Input: part model. Units: mm. Frame: model coordinates. Face numbers are marked on the shaded views. Coordinates: 2 decimals unless noted, no trailing zeros. Order: outer loops, then holes, each group sorted by start corner. A loop starts at its lowest first (then second) coordinate and runs counter-clockwise, first axis right, second up. Notation, with made-up numbers: (-14.75, 82) -> (-3.75, 82) arc R25 cw to (-3.75, 115) -> close; hole circle Ø5 at (28.25, 84). An arc over 180 degrees is marked (long way). Use CSV: the item, a comma, the result in double quotes. Start each with the question number.
```python
from build123d import *

# Parameters (mm, degrees)
SKETCH1_R               = 50.8
BOSS_EXTRUDE1_DEPTH     = 6.35
SKETCH2_R               = 3.175
CUT_EXTRUDE1_DEPTH      = 2.286
SKETCH3_R               = 3.175
CUT_EXTRUDE2_DEPTH      = 1
CUT_EXTRUDE2_DEPTH_BACK = 7.35
SKETCH4_R               = 1.5875
CUT_EXTRUDE3_DEPTH      = 7.35
CHAMFER1_SIZE           = 0.762
FILLET1_R               = 1.27
SKETCH5_R               = 48
SKETCH5_R_2             = 46
BOSS_EXTRUDE2_DEPTH     = 6.35


with BuildPart() as part:
    # Sketch1 → Boss-Extrude1 (new body)
    with BuildSketch(Plane(origin=(0, 0, 0), x_dir=(1, 0, 0), z_dir=(0, 1, 0))):
        Circle(SKETCH1_R)
    extrude(amount=BOSS_EXTRUDE1_DEPTH)

    # Sketch2 → Cut-Extrude1 (cut)
    with BuildSketch(Plane(origin=(0, 6.35, 0), x_dir=(1, 0, 0), z_dir=(0, 1, 0))):
        with Locations((-22.225, -38.494829198)):
            Circle(SKETCH2_R)
        with Locations((-22.225, 38.494829198)):
            Circle(SKETCH2_R)
        with Locations((44.45, 0)):
            Circle(SKETCH2_R)
    extrude(amount=-CUT_EXTRUDE1_DEPTH, mode=Mode.SUBTRACT)

    # Sketch3 → Cut-Extrude2 (cut, two sides)
    with BuildSketch(Plane(origin=(0, 6.35, 0), x_dir=(1, 0, 0), z_dir=(0, 1, 0))) as cut_extrude2_sk:
        Circle(SKETCH3_R)
    extrude(amount=CUT_EXTRUDE2_DEPTH, mode=Mode.SUBTRACT)
    extrude(cut_extrude2_sk.sketch, amount=-CUT_EXTRUDE2_DEPTH_BACK, mode=Mode.SUBTRACT)

    # Sketch4 → Cut-Extrude3 (cut, through all)
    with BuildSketch(Plane.XZ):
        with Locations((50.8, 0)):
            Circle(SKETCH4_R)
        with Locations((-25.4, 43.994090512)):
            Circle(SKETCH4_R)
        with Locations((-25.4, -43.994090512)):
            Circle(SKETCH4_R)
    extrude(amount=-CUT_EXTRUDE3_DEPTH, mode=Mode.SUBTRACT)

    # Chamfer1
    chamfer1_edges = [part.edges().sort_by_distance(p)[0] for p in [
        (25.4, 0, -43.994090512),
        (-50.8, 0, 0),
        (25.4, 0, 43.994090512),
        (25.4, 6.35, -43.994090512),
        (-50.8, 6.35, 0),
        (25.4, 6.35, 43.994090512),
    ]]
    chamfer(chamfer1_edges, length=CHAMFER1_SIZE)

    # Fillet1
    fillet1_edges = [part.edges().sort_by_distance(p)[0] for p in [
        (-24.012950162, 3.175, 44.766262124),
        (-26.76224515, 3.175, 43.178955922),
        (50.775195313, 3.175, -1.587306202),
        (50.775195313, 3.175, 1.587306202),
        (-24.012950162, 3.175, -44.766262124),
        (-26.76224515, 3.175, -43.178955922),
    ]]
    fillet(fillet1_edges, radius=FILLET1_R)

    # Sketch5 → Boss-Extrude2 (add)
    with BuildSketch(Plane.XZ):
        Circle(SKETCH5_R)
        Circle(SKETCH5_R_2, mode=Mode.SUBTRACT)
    extrude(amount=BOSS_EXTRUDE2_DEPTH)


solid = part.part
```
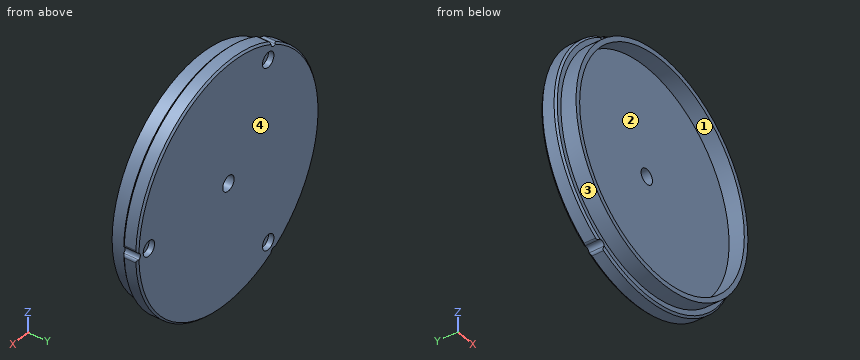
1. Contact query for flat-ended pins moving along their axis: P1, Ø3, axis at x = -22.5, z = 38.5, coming from the +Y side; P2, Ø1.5, axis at y = -1.5, z = 13, coming from the -X side; P3, Ø1.5, axis at x = 3.5, y = 0.5, coming from the +Z side. Output: stop coordinate, or through.
2. Section B-B on x = 0. Return loops of the section in (y, z) (3 decimals).
3. Material intervals for line 1 along X through (y, z) = (4.8, 0) (1 decimal); line 2 along Z through (x, y) = (0, 4.75) (3 decimals); line 3 along X through (y, z) = (5.25, 1.5), sorted ascending.
4. Section C-C on y = -2. Return loops of the section in (x, z).
5. Pull-direction query (Z, two-part tool) for the marked faces 1, 2, 3 and 4; classes: released by +Z, released by -Z, zero draft, split by the parting line, or undercut.
Values follow:
1,P1,"stops at y = 4.06"
1,P2,"stops at x = -46.41"
1,P3,"stops at z = 50.72"
2,outline,"(-6.35, -48) -> (0, -48) -> (0, -50.038) -> (0.762, -50.8) -> (5.588, -50.8) -> (6.35, -50.038) -> (6.35, -3.175) -> (0, -3.175) -> (0, -46) -> (-6.35, -46) -> close; (-6.35, 46) -> (0, 46) -> (0, 3.175) -> (6.35, 3.175) -> (6.35, 50.038) -> (5.588, 50.8) -> (0.762, 50.8) -> (0, 50.038) -> (0, 48) -> (-6.35, 48) -> close"
3,line 1,"x = -50.8 to -3.2, 3.2 to 41.3, 47.6 to 49.2"
3,line 2,"z = -50.8 to -3.175, 3.175 to 50.8"
3,line 3,"x = -50.78 to -2.8, 2.8 to 41.65, 47.25 to 50.21"
4,outline,"circle Ø96 at (0, 0); hole circle Ø92 at (0, 0)"
5,face 1,"undercut"
5,face 2,"undercut"
5,face 3,"split by the parting line"
5,face 4,"zero draft"
